Could you check a few things on this model? Use its own coordinates, in mm. A direction names the side the tool comes from. Round coordinates to 2 decimals unless told otherwise and drop trailing zeros. Loops run counter-clockwise (first coordinate to the right, second up) from the corner with the lowest first, then second, coordinate; pieces in that order, holes last. Notation, with made-up numbers: (65.25, 53) -> (90.25, 53) arc R24 ccw to (90.25, 91) -> close; hole circle Ø5 at (-35.5, 18). An arc over 180 degrees is marked (long way). Write each question's results on one line, items separated by ' | '. Start each with the question number.
1) For P1, Ø2.5, axis at x = 14, y = 14, coming from the +Z side; P2, Ø11.5, axis at x = 0, z = 5.9, coming from the -Y side, each with a flat end and sliding along its axis, tell me the tip position at first contact or that it passes through.
2) If I drill on probe 1 along Y at (x, z) = (-14, 8); probe 2 along X at (y, z) = (12, 2.5); probe 3 along X at (y, z) = (15, -4.75), over which ranges is the centre line in solid material (lowest first)?
3) Imagine slicing it at B-B, the plane x = 14. List the corners of the cut face in (y, z) for me.
4) Which directions (+Z, -Z, +X, -X, +Y, -Y) give clear straight access to the entire face, cutting with the end or side of a thin tool? Please do faces 1 (the flat face through (0, 0, 0)), 2 (the flat face through (0, 4, 0)).
5) Imagine slicing it at D-D, the plane y = 14. List the corners of the cut face in (x, z) for me.
6) Imagine slicing it at A-A, the plane z = 5.9. List the corners of the cut face in (x, y) for me.
7) Imagine slicing it at C-C, the plane y = 3. List the corners of the cut face in (x, z) for me.
8) We'd pull the mould along Y, two halves only. Please class faces 3 (the flat face through (17, 9, 0)), 4 (the flat face through (-14, 18, 0)), 5 (the cylindrical face through (15.5, 14.07, -0.21)): pulls with the +Y half, pulls with the -Y half, needs draft (parallel to the pull), parting line crosses it, or undercut.
from build123d import *

# Parameters (mm, degrees)
SKETCH_1_W          = 34
SKETCH_1_H          = 30
SKETCH_1_R          = 4
SKETCH_1_R_2        = 5
EXTRUDE_1_DEPTH     = 4
SKETCH_3_W          = 6
SKETCH_3_H          = 30
EXTRUDE_2_DEPTH     = 15
SKETCH_4_R          = 1.5
CUT_EXTRUDE_1_DEPTH = 40.37003937
SKETCH_5_W          = 34
SKETCH_5_H          = 1
CUT_EXTRUDE_2_DEPTH = 40.37003937
CHAMFER_1_SIZE      = 1


with BuildPart() as part:
    # 草图1 → 凸台-拉伸1 (new body)
    with BuildSketch(Plane(origin=(0, 0, 0), x_dir=(1, 0, 0), z_dir=(0, 1, 0))):
        Rectangle(SKETCH_1_W, SKETCH_1_H)
        with Locations(Location((0, 6, 0), (0, 0, 270))):
            Circle(SKETCH_1_R, mode=Mode.SUBTRACT)
        with Locations(Location((0, -5.9, 0), (0, 0, 270))):
            Circle(SKETCH_1_R_2, mode=Mode.SUBTRACT)
    extrude(amount=EXTRUDE_1_DEPTH)

    # 草图3 → 凸台-拉伸2 (add)
    with BuildSketch(Plane(origin=(0, 4, 0), x_dir=(1, 0, 0), z_dir=(0, 1, 0))):
        with Locations((-14, 0)):
            Rectangle(SKETCH_3_W, SKETCH_3_H)
        with Locations((14, 0)):
            Rectangle(SKETCH_3_W, SKETCH_3_H)
    extrude(amount=EXTRUDE_2_DEPTH)

    # 草图4 → 切除-拉伸1 (cut, through all)
    with BuildSketch(Plane(origin=(0, 0, -15), x_dir=(-1, 0, 0), z_dir=(0, 0, -1))):
        with Locations((-14, 3)):
            Circle(SKETCH_4_R)
        with Locations((-14, 14)):
            Circle(SKETCH_4_R)
        with Locations(Location((14, 3, 0), (0, 0, 180))):
            Circle(SKETCH_4_R)
        with Locations(Location((14, 14, 0), (0, 0, 180))):
            Circle(SKETCH_4_R)
    extrude(amount=-CUT_EXTRUDE_1_DEPTH, mode=Mode.SUBTRACT)

    # 草图5 → 切除-拉伸2 (cut, through all)
    with BuildSketch(Plane(origin=(0, 0, -15), x_dir=(-1, 0, 0), z_dir=(0, 0, -1))):
        with Locations((0, 18.5)):
            Rectangle(SKETCH_5_W, SKETCH_5_H)
    extrude(amount=-CUT_EXTRUDE_2_DEPTH, mode=Mode.SUBTRACT)

    # 倒角1
    chamfer_1_edges = [part.edges().sort_by_distance(p)[0] for p in [
        (0, 0, -10),
    ]]
    chamfer(chamfer_1_edges, length=CHAMFER_1_SIZE)


solid = part.part
Checked values:
1) P1: through | P2: y = 0
2) probe 1: 0 to 1.5, 4.5 to 12.5, 15.5 to 18 | probe 2: -17 to -11, 11 to 17 | probe 3: -17 to -15.12, -12.88 to -11, 11 to 12.88, 15.12 to 17
3) outline: (0, -15) -> (1.5, -15) -> (1.5, 15) -> (0, 15) -> close; (4.5, -15) -> (12.5, -15) -> (12.5, 15) -> (4.5, 15) -> close; (15.5, -15) -> (18, -15) -> (18, 15) -> (15.5, 15) -> close
4) face 1: +Z, -Z, +X, -X, -Y | face 2: +Z, -Z, +Y
5) outline: (-17, -15) -> (-15.5, -15) -> (-15.5, 15) -> (-17, 15) -> close; (-12.5, -15) -> (-11, -15) -> (-11, 15) -> (-12.5, 15) -> close; (11, -15) -> (12.5, -15) -> (12.5, 15) -> (11, 15) -> close; (15.5, -15) -> (17, -15) -> (17, 15) -> (15.5, 15) -> close
6) outline: (-17, 0) -> (-5, 0) -> (-5, 4) -> (-11, 4) -> (-11, 18) -> (-17, 18) -> close; (5, 0) -> (17, 0) -> (17, 18) -> (11, 18) -> (11, 4) -> (5, 4) -> close; hole circle Ø3 at (-14, 3); hole circle Ø3 at (-14, 14); hole circle Ø3 at (14, 3); hole circle Ø3 at (14, 14)
7) outline: (-17, -15) -> (-15.5, -15) -> (-15.5, 15) -> (-17, 15) -> close; (-12.5, -15) -> (12.5, -15) -> (12.5, 15) -> (-12.5, 15) -> close; (15.5, -15) -> (17, -15) -> (17, 15) -> (15.5, 15) -> close; hole circle Ø10 at (0, 5.9); hole circle Ø8 at (0, -6)
8) face 3: needs draft | face 4: pulls with the +Y half | face 5: undercut
